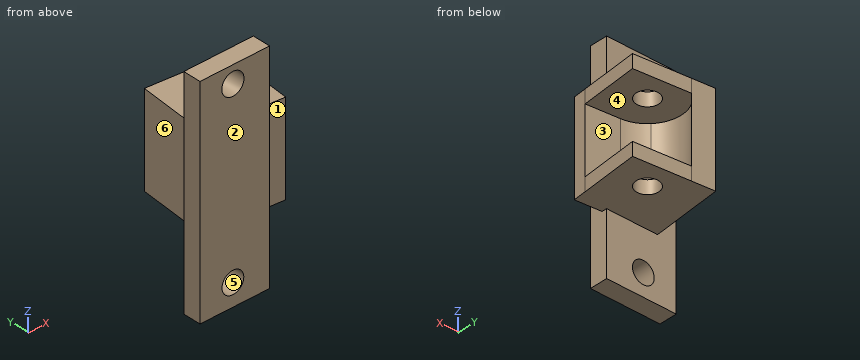
from build123d import *

# Parameters (mm, degrees)
BOSS_EXTRUDE1_DEPTH = 22.352
BOSS_EXTRUDE2_START = -3.81
SKETCH2_R           = 3.175
BOSS_EXTRUDE2_DEPTH = 3.81
BOSS_EXTRUDE4_START = 3.81
SKETCH3_R           = 3.175
BOSS_EXTRUDE4_DEPTH = 3.81
SKETCH4_W           = 19.88678917
SKETCH4_H           = 61.722
BOSS_EXTRUDE5_DEPTH = 5.08
SKETCH6_R           = 3.175
SKETCH6_R_2         = 3.112599105
CUT_EXTRUDE2_DEPTH  = 5.08


with BuildPart() as part:
    # Sketch1 → Boss-Extrude1 (new body)
    with BuildSketch(Plane.XY):
        with BuildLine():
            Line((-476.384421201, 136.819327006), (-476.01254536, 140.611135065))
            Line((-476.01254536, 140.611135065), (-485.284620904, 141.520479852))
            ThreePointArc((-485.284620904, 141.520479852), (-488.563156596, 142.455032775), (-491.302607825, 144.484217934))
            ThreePointArc((-491.302607825, 144.484217934), (-493.83445145, 151.929689602), (-489.904354663, 158.741416237))
            Line((-489.904354663, 158.741416237), (-496.224034762, 159.361209305))
            Line((-496.224034762, 159.361209305), (-498.224726786, 138.961281946))
            Line((-498.224726786, 138.961281946), (-476.384421201, 136.819327006))
        make_face()
    extrude(amount=-BOSS_EXTRUDE1_DEPTH)

    # Sketch2 → Boss-Extrude2 (add)
    with BuildSketch(Plane(origin=(0, 0, -22.352), x_dir=(-1, 0, 0), z_dir=(0, 0, -1)).offset(BOSS_EXTRUDE2_START)):
        with BuildLine():
            Line((474.383729176, 157.219254365), (489.904354663, 158.741416237))
            ThreePointArc((489.904354663, 158.741416237), (493.55465351, 148.532058286), (485.284620904, 141.520479852))
            Line((485.284620904, 141.520479852), (476.01254536, 140.611135065))
            Line((476.01254536, 140.611135065), (474.383729176, 157.219254365))
        make_face()
        with Locations((484.354931302, 151)):
            Circle(SKETCH2_R, mode=Mode.SUBTRACT)
    extrude(amount=BOSS_EXTRUDE2_DEPTH)

    # Sketch3 → Boss-Extrude4 (add)
    # profile 1 of 2: a face of its own
    with BuildSketch(Plane.XY.offset(BOSS_EXTRUDE4_START)):
        with BuildLine():
            Line((-474.383729176, 157.219254365), (-489.904354663, 158.741416237))
            ThreePointArc((-489.904354663, 158.741416237), (-493.55465351, 148.532058286), (-485.284620904, 141.520479852))
            Line((-485.284620904, 141.520479852), (-476.01254536, 140.611135065))
            Line((-476.01254536, 140.611135065), (-474.383729176, 157.219254365))
        make_face()
        with Locations(Location((-484.354931302, 151, 0), (0, 0, 180))):
            Circle(SKETCH3_R, mode=Mode.SUBTRACT)
    # profile 2 of 2: a face of its own
    with BuildSketch(Plane.XY.offset(BOSS_EXTRUDE4_START)):
        with BuildLine():
            Line((-476.01254536, 140.611135065), (-485.284620904, 141.520479852))
            ThreePointArc((-485.284620904, 141.520479852), (-493.55465351, 148.532058286), (-489.904354663, 158.741416237))
            Line((-489.904354663, 158.741416237), (-496.224034762, 159.361209305))
            Line((-496.224034762, 159.361209305), (-498.224726786, 138.961281946))
            Line((-498.224726786, 138.961281946), (-476.384421201, 136.819327006))
            Line((-476.384421201, 136.819327006), (-476.01254536, 140.611135065))
        make_face()
    extrude(amount=-BOSS_EXTRUDE4_DEPTH)

    # Sketch4 → Boss-Extrude5 (add)
    with BuildSketch(Plane(origin=(0, 138.961281946, 0), x_dir=(1, 0, 0), z_dir=(0, 1, 0))):
        with Locations((-493.624258186, 9.271)):
            Rectangle(SKETCH4_W, SKETCH4_H)
    extrude(amount=-BOSS_EXTRUDE5_DEPTH)

    # Sketch6 → Cut-Extrude2 (cut)
    with BuildSketch(Plane(origin=(0, 138.961281946, 0), x_dir=(1, 0, 0), z_dir=(0, 1, 0))):
        with Locations(Location((-494.169652771, -16.705193035, 0), (0, 0, 270))):
            Circle(SKETCH6_R)
        with Locations(Location((-494.169652771, 33.836204424, 0), (0, 0, 270))):
            Circle(SKETCH6_R_2)
    extrude(amount=-CUT_EXTRUDE2_DEPTH, mode=Mode.SUBTRACT)


solid = part.part
Model file for the job. Use its own axes, mm. Face numbers are marked on the shaded views. A direction names the side the tool comes from. Give positions to 0.01 mm unless a question says otherwise; leave off trailing zeros. Order: outer loops, then holes, each group sorted by start corner. A loop starts at its lowest first (then second) coordinate and runs counter-clockwise, first axis right, second up. Notation, with made-up numbers: (-22, 18) - (-8, 18) arc R23 cw to (-8, 51) - close; hole circle Ø8 at (-28.5, 44.5). An arc over 180 degrees is marked (long way). Return JSON: item names as keys, results as strings.
1) 3-axis set-ups, long thin cutter, end or side, ignore diameter. For the marked faces 1, 2 and 3: which of +Z, -Z, +X, -X, +Y, -Y reach the whole face in a straight line?
Geometry says:
{"face 1": "+Z, -Z, -Y", "face 2": "+Z, -Z, +X, -X, -Y", "face 3": "+X, +Y"}
2) Cut at D-D, the plane z = -7.5. Give the cut face in (x, y) (3 decimals).
Geometry says:
{"outline": "(-503.568, 133.881) - (-483.681, 133.881) - (-483.681, 137.535) - (-476.384, 136.819) - (-476.013, 140.611) - (-485.285, 141.52) arc R9.525 cw to (-489.904, 158.741) - (-496.224, 159.361) - (-498.225, 138.961) - (-503.568, 138.961) - close"}
3) Probe line 1 (Z direction, x = -492.5, y = 138.5); line 2 (Z direction, x = -475.75, y = 148.5); line 3 (Z direction, x = -493.25, y = 138). List the from-to ranges inside material, lowest first. Write a range as from..to.
Geometry says:
{"line 1": "-40.13..-36.46, -31.21..14, 19.41..21.59", "line 2": "-22.35..-18.54, 0..3.81", "line 3": "-40.13..-36.81, -30.86..13.67, 19.74..21.59"}
4) Cut at A-A, the plane z = -20. Give the cut face in (x, y) (3 decimals), plus the area to 3 significant figures.
Geometry says:
{"outline": "(-503.568, 133.881) - (-483.681, 133.881) - (-483.681, 137.535) - (-476.384, 136.819) - (-474.384, 157.219) - (-496.224, 159.361) - (-498.225, 138.961) - (-503.568, 138.961) - close; hole circle Ø6.35 at (-484.355, 151)", "area": "509 mm²"}
5) Cut at C-C, the plane x = -486.5. Give the cut face in (y, z), plus the area to 3 significant figures.
Geometry says:
{"outline": "(133.88, -40.13) - (138.96, -40.13) - (138.96, -22.35) - (148.66, -22.35) - (148.66, -18.54) - (141.72, -18.54) - (141.72, 0) - (148.66, 0) - (148.66, 3.81) - (138.96, 3.81) - (138.96, 21.59) - (133.88, 21.59) - close; (153.34, -22.35) - (158.41, -22.35) - (158.41, -18.54) - (153.34, -18.54) - close; (153.34, 0) - (158.41, 0) - (158.41, 3.81) - (153.34, 3.81) - close", "area": "477 mm²"}
6) Cut at B-B, the plane y = 151. Give the cut face in (x, z), plus the area to 3 significant figures.
Geometry says:
{"outline": "(-497.04, -22.35) - (-487.53, -22.35) - (-487.53, -18.54) - (-493.88, -18.54) - (-493.88, 0) - (-487.53, 0) - (-487.53, 3.81) - (-497.04, 3.81) - close; (-481.18, -22.35) - (-474.99, -22.35) - (-474.99, -18.54) - (-481.18, -18.54) - close; (-481.18, 0) - (-474.99, 0) - (-474.99, 3.81) - (-481.18, 3.81) - close", "area": "178 mm²"}
7) Pull direction Y, two halves, no side cores. Call the marked faces 4, 5 and 6: pulls with the +Y half, pulls with the -Y half, needs draft (parallel to the pull), parting line crosses it, or undercut.
Geometry says:
{"face 4": "undercut", "face 5": "needs draft", "face 6": "pulls with the +Y half"}
8) Flat gauge pins, fed straight in: P1, Ø9, axis at x = -485.5, y = 152.5, coming from the -Z side; P2, Ø10, axis at y = 155, z = 6, coming from the -X side; P3, Ø3, axis at y = 146.5, z = -16, coming from the +X side; P4, Ø5, axis at x = -494.17, z = 16.71, coming from the -Y side. Where does each tip first touch, or does it go through?
Geometry says:
{"P1": "z = -22.35", "P2": "x = -497.09", "P3": "x = -491.75", "P4": "through"}
